```python
from build123d import *

# Parameters (mm, degrees)
TAP_DRILL_FOR_1_4_TAP_1_4_18_NPT_D                   = 11.1252
CBORE_FOR_1_4_BINDING_HEAD_MACHINE_SCREW_D           = 6.7564
CBORE_FOR_1_4_BINDING_HEAD_MACHINE_SCREW_CBORE_D     = 12.7
CBORE_FOR_1_4_BINDING_HEAD_MACHINE_SCREW_CBORE_DEPTH = 3.81


with BuildPart() as part:
    # Sketch1 → Revolve1 (revolve)
    with BuildSketch(Plane.XY, mode=Mode.PRIVATE) as revolve1_sk:
        Polygon((0, 0), (47.498, 0), (47.498, 2.4638), (44.577, 2.4638), (44.577, 7.4422), (47.498, 7.4422), (47.498, 9.906), (41.148, 9.906), (41.148, 6.35), (0, 6.35), align=None)
    revolve(revolve1_sk.sketch.rotate(Axis((0, 48.192213231, 0), (0, -1, 0)), 180), axis=Axis((0, 48.192213231, 0), (0, -1, 0)))

    # Tap Drill for 1/4 Tap - 1/4-18 NPT (through all)
    with Locations(Plane(origin=(0, 6.35, 0), x_dir=(1, 0, 0), z_dir=(0, 1, 0))):
        with Locations((-30.1752, 0)):
            Hole(TAP_DRILL_FOR_1_4_TAP_1_4_18_NPT_D / 2)

    # CBORE for 1/4 Binding Head Machine Screw1 (through all)
    with Locations(Plane.XZ):
        with Locations((12.150198978, -29.333175157), (-12.150198978, 29.333175157)):
            CounterBoreHole(CBORE_FOR_1_4_BINDING_HEAD_MACHINE_SCREW_D / 2, CBORE_FOR_1_4_BINDING_HEAD_MACHINE_SCREW_CBORE_D / 2, CBORE_FOR_1_4_BINDING_HEAD_MACHINE_SCREW_CBORE_DEPTH)


solid = part.part
```
Source: CAD feature listing. Evaluate the final solid. Frame: model axes, mm. A direction names the side the tool comes from. Round coordinates to 2 decimals unless told otherwise and drop trailing zeros. Loops run counter-clockwise (first coordinate to the right, second up) from the corner with the lowest first, then second, coordinate; pieces in that order, holes last. Notation, with made-up numbers: M 48.5,84.5 L 87.5,84.5 A13 cw 87.5,93.5 Z; hole C 46.5,27 d10. An arc over 180 degrees is marked long. Use a Markdown table: item, result. Add a question column.
1. Cut plane B-B, the plane x = 0. Output: boundary loops of the cut face in (y, z), and give its area (3 significant figures).
2. Cut plane C-C, the plane y = 5.25. Output: boundary loops of the cut face in (x, z), and give its area (3 significant figures).
3. Contact query for flat-ended pins moving along their axis: pin 1 (3 mm diameter, centred on x = 14.5, y = 7.5, fed in from -Z); pin 2 (6 mm diameter, centred on x = 12.15, z = -29.33, fed in from -Y); pin 3 (14.5 mm diameter, centred on x = -12.15, z = 29.33, fed in from +Y); pin 4 (2 mm diameter, centred on y = 8, z = 26, fed in from +X). Output: stop coordinate, or through.
4. Cut plane A-A, the plane z = 0. Output: boundary loops of the cut face in (x, y), and give its area (3 significant figures).
5. Cut plane D-D, the plane z = -10.5. Output: boundary loops of the cut face in (x, y), and give its area (3 significant figures).
6. Set-up query: faces 4 (the flat face through (-14.3, 7.442, -42.4)), 5 (the flat face through (-9, 3.81, 27)), 6 (the flat face through (1, 6.35, -1)), 7 (the cylindrical face through (-45.305, 1.249, -14.267)). Return all of +Z, -Z, +X, -X, +Y, -Y with unobstructed straight access to the full face (end or side cutting, diameter ignored); none if empty.
7. Pull-direction query (Z, two-part tool) for faces 1 (the cylindrical face through (7.111, 1.878, -33.197)), 2 (the cylindrical face through (32.855, 4.988, -30.127)), 3 (the flat face through (-1, 0, -1)); classes: +Z half, -Z half, draft (parallel to the pull), parting line (faces both ways), or undercut.
8. Ray query, line 1 along Z through (x, y) = (1, 8.5); line 2 along Y through (x, z) = (-6, 7); line 3 along X through (y, z) = (4.25, -0.5). Return the intervals inside material, ascending. Write a range as [from, to].
Solution:
| question | item | result |
|---|---|---|
| 1 | outline | M 0,-47.5 L 2.46,-47.5 L 2.46,-44.58 L 7.44,-44.58 L 7.44,-47.5 L 9.91,-47.5 L 9.91,-41.15 L 6.35,-41.15 L 6.35,41.15 L 9.91,41.15 L 9.91,47.5 L 7.44,47.5 L 7.44,44.58 L 2.46,44.58 L 2.46,47.5 L 0,47.5 Z |
| 1 | area | 619 mm2 |
| 2 | outline | C 0,0 d89.15; hole C -30.18,0 d11.13; hole C -12.15,29.33 d6.76; hole C 12.15,-29.33 d6.76 |
| 2 | area | 6,070 mm2 |
| 3 | pin 1 | stops at z = -45.68 |
| 3 | pin 2 | passes through |
| 3 | pin 3 | stops at y = 6.35 |
| 3 | pin 4 | stops at x = 40.39 |
| 4 | outline | M -47.5,0 L -35.74,0 L -35.74,6.35 L -41.15,6.35 L -41.15,9.91 L -47.5,9.91 L -47.5,7.44 L -44.58,7.44 L -44.58,2.46 L -47.5,2.46 Z; M -24.61,0 L 47.5,0 L 47.5,2.46 L 44.58,2.46 L 44.58,7.44 L 47.5,7.44 L 47.5,9.91 L 41.15,9.91 L 41.15,6.35 L -24.61,6.35 Z |
| 4 | area | 549 mm2 |
| 5 | outline | M -46.32,0 L 46.32,0 L 46.32,2.46 L 43.32,2.46 L 43.32,7.44 L 46.32,7.44 L 46.32,9.91 L 39.79,9.91 L 39.79,6.35 L -39.79,6.35 L -39.79,9.91 L -46.32,9.91 L -46.32,7.44 L -43.32,7.44 L -43.32,2.46 L -46.32,2.46 Z |
| 5 | area | 605 mm2 |
| 6 | face 4 | none |
| 6 | face 5 | -Y |
| 6 | face 6 | +Y |
| 6 | face 7 | +Y, -Y |
| 7 | face 1 | undercut |
| 7 | face 2 | parting line |
| 7 | face 3 | draft |
| 8 | line 1 | z = [-47.49, -41.14], [41.14, 47.49] |
| 8 | line 2 | y = [0, 6.35] |
| 8 | line 3 | x = [-44.57, -35.72], [-24.64, 44.57] |
